Source: CAD feature listing. Evaluate the final solid. Frame: model axes, mm. Coordinates: 2 decimals unless noted, no trailing zeros. Write each loop counter-clockwise with the first axis right and the second up, starting at its lowest first coordinate (ties: lowest second). Pieces come first, ordered by that corner, then holes. Notation, with made-up numbers: (66.25, -22) -> (117.25, -22) arc R35 ccw to (117.25, 11) -> close; hole circle Ø10 at (17, -25). An arc over 180 degrees is marked (long way). One line per item, written item: value. Start each with the question number.
1. Section query B-B, the plane y = -16.5. Output: boundary loops of the cut face in (x, z).
2. Section query A-A, the plane x = -6. Output: boundary loops of the cut face in (y, z), and give its area (3 significant figures).
3. Line query: line 1 (Y direction, x = -4, z = 2.7); line 2 (X direction, y = -6.5, z = 1.4). Output: solid intervals per line, ascending.
4. Section query C-C, the plane z = 2.1. Output: boundary loops of the cut face in (x, y), and give its area (3 significant figures).
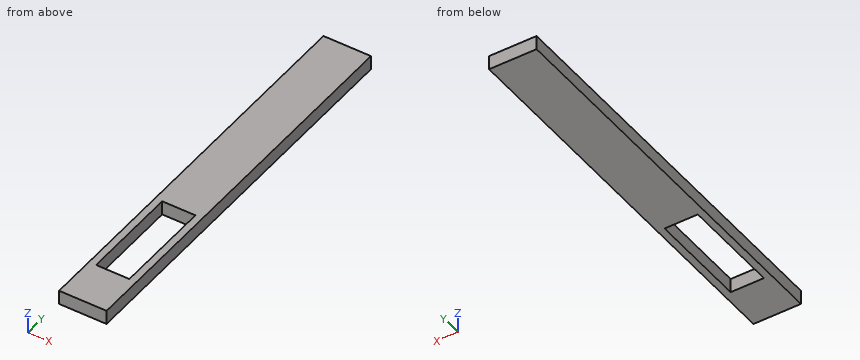
from build123d import *

# Parameters (mm, degrees)
ESBO_O1_W                = 10
ESBO_O1_H                = 9
ESBO_O1_H_2              = 66
ESBO_O1_W_2              = 7
ESBO_O1_H_3              = 21
RESSALTO_EXTRUS_O1_DEPTH = 3


with BuildPart() as part:
    # Esboço1 → Ressalto-extrusão1 (new body)
    with BuildSketch(Plane.XY):
        with Locations((-4.707063062, 47.072338936)):
            Rectangle(ESBO_O1_W, ESBO_O1_H)
        with Locations((-4.707063062, 9.572338936)):
            Rectangle(ESBO_O1_W, ESBO_O1_H_2)
        with Locations((-4.707063062, -12.427661064)):
            Rectangle(ESBO_O1_W_2, ESBO_O1_H_3, mode=Mode.SUBTRACT)
        with Locations((-4.707063062, -27.927661064)):
            Rectangle(ESBO_O1_W, ESBO_O1_H)
    extrude(amount=RESSALTO_EXTRUS_O1_DEPTH)


solid = part.part
Computed values:
1. outline: (-9.71, 0) -> (-8.21, 0) -> (-8.21, 3) -> (-9.71, 3) -> close; (-1.21, 0) -> (0.29, 0) -> (0.29, 3) -> (-1.21, 3) -> close
2. outline: (-32.43, 0) -> (-22.93, 0) -> (-22.93, 3) -> (-32.43, 3) -> close; (-1.93, 0) -> (51.57, 0) -> (51.57, 3) -> (-1.93, 3) -> close
2. area: 189 mm²
3. line 1: y = -32.43 to -22.93, -1.93 to 51.57
3. line 2: x = -9.71 to -8.21, -1.21 to 0.29
4. outline: (-9.71, -32.43) -> (0.29, -32.43) -> (0.29, 51.57) -> (-9.71, 51.57) -> close; hole (-8.21, -22.93) -> (-1.21, -22.93) -> (-1.21, -1.93) -> (-8.21, -1.93) -> close
4. area: 693 mm²
